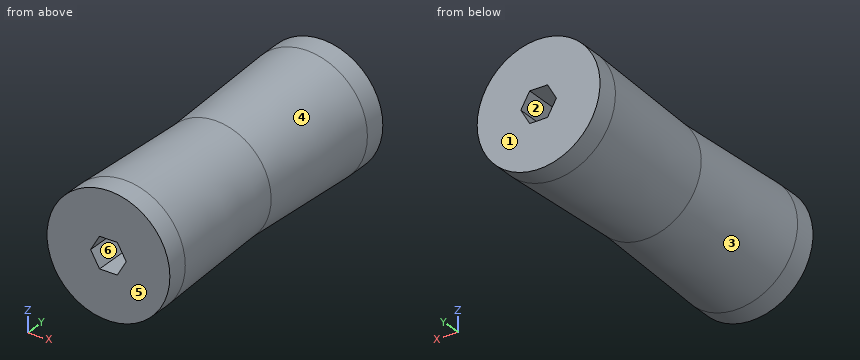
```python
from build123d import *

# Parameters (mm, degrees)
F0_R     = 25.4
F1_DEPTH = 63.5


with BuildPart() as f1:
    # F0 (on Front) → F1 (new body)
    with BuildSketch(Plane.XZ):
        Circle(F0_R)
        Polygon((7.361678, 0), (3.680839, -6.3754), (-3.680839, -6.3754), (-7.361678, 0), (-3.680839, 6.3754), (3.680839, 6.3754), align=None, mode=Mode.SUBTRACT)
    extrude(amount=F1_DEPTH)

    # F2 (on Right) → F3 (revolve, cut)
    with BuildSketch(Plane.YZ):
        Polygon((-63.5, 25.606239), (-63.5, 23.248794), (-3.98305, 25.606239), align=None)
    revolve(axis=Axis((0, -31.75, 0), (0, -1, 0)), mode=Mode.SUBTRACT)

    # F5: F1 across plane


with BuildPart() as f1_1:
    add(f1.part)
    add(f1.part.mirror(Plane.XZ.offset(63.5)))


solid = f1_1.part
```
Check sheet for the modelled part. Datum: model origin and axes. Units: mm. Face numbers are marked on the shaded views. A direction names the side the tool comes from. Round coordinates to 2 decimals unless told otherwise and drop trailing zeros. Loops run counter-clockwise (first coordinate to the right, second up) from the corner with the lowest first, then second, coordinate; pieces in that order, holes last. Notation, with made-up numbers: (-18.75, -8.5) - (-9.75, -8.5) arc R21 cw to (-9.75, 0.5) - close; hole circle Ø5 at (36, -35.5). An arc over 180 degrees is marked (long way). Answer as a JSON object with one key per item and string values. Group by question number.
Q1. Set-up check for the marked faces 5 and 6: record each of +Z, -Z, +X, -X, +Y, -Y from which the full face is reachable in a straight line by a thin tool's end or side.
Q2. Sectioned sample at A-A, the plane y = -45.5. Enter the section's corners in (x, z).
Q3. Mould release check, pull along Y, two halves, no side actions. Record for the marked faces 1, 2, 3 and 4: released by +Y, released by -Y, zero draft, split by the parting line, or undercut.
Q4. Gauge pin test, flat ends, axial feed: P1, Ø10, axis at x = 6, y = -85, coming from the -Z side; P2, Ø10, axis at y = -59.5, z = 6.5, coming from the +X side; P3, Ø3.5, axis at x = 0.5, y = -58.5, coming from the -Z side; P4, Ø3, axis at x = 10, z = 16.5, coming from the +Y side. Record the tip position at first contact, or that the pin passes through.
Q5. Scan lines: line 1 along X through (y, z) = (-17.5, -1); line 2 along Z through (x, y) = (-5, -79); line 3 along Z through (x, y) = (5.5, -80.5). Record each from-to range of solid material in increasing order. Write a range as [from, to].
Q6. Sectioned sample at B-B, the plane x = 0. Enter the section's corners in (y, z).
Solution:
{
 "1": {"face 5": "+Z, -Z, +X, -X, -Y", "face 6": "+Y, -Y"},
 "2": {"outline": "circle Ø47.92 at (0, 0); hole (-7.36, 0) - (-3.68, -6.38) - (3.68, -6.38) - (7.36, 0) - (3.68, 6.38) - (-3.68, 6.38) - close"},
 "3": {"face 1": "released by +Y", "face 2": "zero draft", "face 3": "undercut", "face 4": "undercut"},
 "4": {"P1": "stops at z = -24.14", "P2": "stops at x = 23.41", "P3": "stops at z = -23.51", "P4": "stops at y = 0"},
 "5": {"line 1": "x = [-25.05, -6.78], [6.78, 25.05]", "line 2": "z = [-23.33, -4.09], [4.09, 23.33]", "line 3": "z = [-23.28, -3.22], [3.22, 23.28]"},
 "6": {"outline": "(-127, -25.4) - (-117.81, -25.4) - (-63.5, -23.25) - (-9.19, -25.4) - (0, -25.4) - (0, -6.38) - (-127, -6.38) - close; (-127, 6.38) - (0, 6.38) - (0, 25.4) - (-9.19, 25.4) - (-63.5, 23.25) - (-117.81, 25.4) - (-127, 25.4) - close"}
}
